Verification items for the finished model (mm, model axes). A direction names the side the tool comes from. Coordinates: 2 decimals unless noted, no trailing zeros. Order: outer loops, then holes, each group sorted by start corner. A loop starts at its lowest first (then second) coordinate and runs counter-clockwise, first axis right, second up. Notation, with made-up numbers: (57.5, 16) -> (81.5, 16) arc R19 ccw to (81.5, 34) -> close; hole circle Ø4 at (26, 38.5). An arc over 180 degrees is marked (long way). Answer as CSV lines item,"result".
```python
from build123d import *

# Parameters (mm, degrees)
EXTRUDE_1_DEPTH          = 5
SKETCH_2_W               = 4
SKETCH_2_H               = 40
EXTRUDE_2_DEPTH          = 36
EXTRUDE_3_DEPTH          = 7.5
CUT_EXTRUDE_2_DEPTH      = 14
EXTRUDE_START            = 18
SKETCH_5_W               = 5
SKETCH_5_H               = 27.5
EXTRUDE_4_DEPTH          = 18
SKETCH_6_R               = 15
SKETCH_6_R_2             = 1.5
CUT_EXTRUDE_3_DEPTH      = 18
CUT_EXTRUDE_4_DEPTH      = 15
CUT_EXTRUDE_4_DEPTH_BACK = 26
SKETCH_9_R               = 1.65
CUT_EXTRUDE_5_DEPTH      = 41
RIB_2_REACH              = 138.99
SKETCH_10_WALL_W         = 293.529278964
SKETCH_10_WALL_H         = 10
EXTRUDE_6_DEPTH          = 5
SKETCH_12_W              = 36
SKETCH_12_H              = 5
CUT_EXTRUDE_6_DEPTH      = 87


with BuildPart() as part:
    # 草图1 → 凸台-拉伸1 (new body)
    with BuildSketch(Plane.XY):
        with BuildLine():
            Line((105.214975384, -55), (105.214975384, 50))
            Line((105.214975384, 50), (-51, 50))
            ThreePointArc((-51, 50), (-53.828427125, 48.828427125), (-55, 46))
            Line((-55, 46), (-55, -46))
            ThreePointArc((-55, -46), (-53.828427125, -48.828427125), (-51, -50))
            Line((-51, -50), (-49.468062182, -50))
            Line((-49.468062182, -50), (-49.468062182, -55))
            Line((-49.468062182, -55), (-39.468062182, -55))
            Line((-39.468062182, -55), (-39.468062182, -50))
            Line((-39.468062182, -50), (35.214975384, -50))
            Line((35.214975384, -50), (35.214975384, -55))
            Line((35.214975384, -55), (105.214975384, -55))
        make_face()
    extrude(amount=EXTRUDE_1_DEPTH)

    # 草图2 → 凸台-拉伸2 (add)
    with BuildSketch(Plane(origin=(0, 0, 0), x_dir=(-1, 0, 0), z_dir=(0, 0, -1))):
        with Locations((35, 21.933022766)):
            Rectangle(SKETCH_2_W, SKETCH_2_H)
        with Locations((-1, 21.933022766)):
            Rectangle(SKETCH_2_W, SKETCH_2_H)
        with Locations((-18, 21.933022766)):
            Rectangle(SKETCH_2_W, SKETCH_2_H)
    extrude(amount=EXTRUDE_2_DEPTH)

    # 草图3 → 凸台-拉伸3 (add, symmetric)
    with BuildSketch(Plane(origin=(0, 20, 0), x_dir=(1, 0, 0), z_dir=(0, 1, 0))):
        Polygon((20, 12.468062182), (20, 0), (30.673808223, 0), align=None)
        Polygon((16, 12.468062182), (9.436406156, 0), (16, 0), align=None)
        Polygon((3, 12.468062182), (3, 0), (9.436406156, 0), align=None)
        Polygon((-1, 12.468062182), (-8.755927232, 0), (-1, 0), align=None)
        Polygon((-33, 12.468062182), (-33, 0), (-24.531937818, 0), align=None)
        Polygon((-37, 12.468062182), (-49.468062182, 0), (-37, 0), align=None)
    extrude(amount=EXTRUDE_3_DEPTH, both=True)

    # 草图4 → 切除-拉伸2 (cut)
    with BuildSketch(Plane(origin=(0, 0, 0), x_dir=(-1, 0, 0), z_dir=(0, 0, -1))):
        with BuildLine():
            Line((18.5, -18.5), (18.5, -36))
            ThreePointArc((18.5, -36), (19.671572875, -38.828427125), (22.5, -40))
            Line((22.5, -40), (48, -40))
            ThreePointArc((48, -40), (50.121320344, -39.121320344), (51, -37))
            Line((51, -37), (51, -17.5))
            ThreePointArc((51, -17.5), (50.121320344, -15.378679656), (48, -14.5))
            Line((48, -14.5), (22.5, -14.5))
            ThreePointArc((22.5, -14.5), (19.671572875, -15.671572875), (18.5, -18.5))
        make_face()
    extrude(amount=-CUT_EXTRUDE_2_DEPTH, mode=Mode.SUBTRACT)

    # 草图5 → 凸台-拉伸4 (add)
    with BuildSketch(Plane(origin=(0, 0, 0), x_dir=(-1, 0, 0), z_dir=(0, 0, -1)).offset(EXTRUDE_START)):
        with Locations((-43.5, -27.25)):
            Rectangle(SKETCH_5_W, SKETCH_5_H)
        with BuildLine():
            Line((18.5, -18.5), (18.5, -36))
            ThreePointArc((18.5, -36), (19.671572875, -38.828427125), (22.5, -40))
            Line((22.5, -40), (48, -40))
            Line((48, -40), (48, -44))
            Line((48, -44), (11.223006292, -44))
            Line((11.223006292, -44), (11.223006292, -41))
            Line((11.223006292, -41), (11.223006292, -13.5))
            Line((11.223006292, -13.5), (11.223006292, -10.5))
            Line((11.223006292, -10.5), (48, -10.5))
            Line((48, -10.5), (48, -14.5))
            Line((48, -14.5), (22.5, -14.5))
            ThreePointArc((22.5, -14.5), (19.671572875, -15.671572875), (18.5, -18.5))
        make_face()
    extrude(amount=-EXTRUDE_4_DEPTH)

    # 草图6 → 切除-拉伸3 (cut)
    with BuildSketch(Plane(origin=(0, 0, 0), x_dir=(-1, 0, 0), z_dir=(0, 0, -1))):
        with Locations((-11.776993708, -27.5)):
            Circle(SKETCH_6_R)
        with Locations((4.223006292, -43.5)):
            Circle(SKETCH_6_R_2)
        with Locations((4.223006292, -11.5)):
            Circle(SKETCH_6_R_2)
        with Locations((-27.776993708, -11.5)):
            Circle(SKETCH_6_R_2)
        with Locations((-27.776993708, -43.5)):
            Circle(SKETCH_6_R_2)
    extrude(amount=-CUT_EXTRUDE_3_DEPTH, mode=Mode.SUBTRACT)

    # 草图7 → 切除-拉伸4 (cut, two sides: drawn at the far end of the back side and taken through both)
    with BuildSketch(Plane.XY.offset(5).offset(-CUT_EXTRUDE_4_DEPTH_BACK)):
        with BuildLine():
            Line((78.295417345, 28.5), (87.295417345, 28.5))
            ThreePointArc((87.295417345, 28.5), (88.709630907, 29.085786438), (89.295417345, 30.5))
            Line((89.295417345, 30.5), (89.295417345, 32.5))
            ThreePointArc((89.295417345, 32.5), (88.709630907, 33.914213562), (87.295417345, 34.5))
            Line((87.295417345, 34.5), (78.295417345, 34.5))
            ThreePointArc((78.295417345, 34.5), (76.881203783, 33.914213562), (76.295417345, 32.5))
            Line((76.295417345, 32.5), (76.295417345, 30.5))
            ThreePointArc((76.295417345, 30.5), (76.881203783, 29.085786438), (78.295417345, 28.5))
        make_face()
    extrude(amount=CUT_EXTRUDE_4_DEPTH + CUT_EXTRUDE_4_DEPTH_BACK, mode=Mode.SUBTRACT)

    # 草图9 → 切除-拉伸5 (cut)
    with BuildSketch(Plane.XY.offset(5)):
        with Locations((-44.468062182, -50.360148647)):
            Circle(SKETCH_9_R)
        with Locations((-51.519821375, 46.879485601)):
            Circle(SKETCH_9_R)
        with Locations((60.214975384, -48.977955399)):
            Circle(SKETCH_9_R)
        with Locations((59.391625653, 46)):
            Circle(SKETCH_9_R)
        with Locations((98.214975384, -48.977955399)):
            Circle(SKETCH_9_R)
        with Locations((94.391625653, 46)):
            Circle(SKETCH_9_R)
    extrude(amount=-CUT_EXTRUDE_5_DEPTH, mode=Mode.SUBTRACT)

    # 草图10 wall → 筋2 (add, up to next)
    with BuildSketch(Plane(origin=(50.748705284, -30, -7.378924001), x_dir=(0.541169685132, 0, 0.840913415218), z_dir=(0.840913415218, 0, -0.541169685132)), mode=Mode.PRIVATE) as rib_2_sk1:
        Rectangle(SKETCH_10_WALL_W, SKETCH_10_WALL_H)
    rib_2_tool1 = extrude(rib_2_sk1.sketch, amount=-RIB_2_REACH, mode=Mode.PRIVATE) - part.part
    add(rib_2_tool1.solids().sort_by_distance((50.748705284, -30, -7.378924001))[0])

    # 草图11 → 凸台-拉伸6 (add)
    with BuildSketch(Plane(origin=(46, 0, 0), x_dir=(0, 0, -1), z_dir=(1, 0, 0))):
        Polygon((18, -13.5), (0, -4.773458624), (0, -13.5), align=None)
    extrude(amount=-EXTRUDE_6_DEPTH)

    # 草图12 → 切除-拉伸6 (cut)
    with BuildSketch(Plane(origin=(20, 0, 0), x_dir=(0, 0, -1), z_dir=(1, 0, 0))):
        with Locations((18, 4.433022766)):
            Rectangle(SKETCH_12_W, SKETCH_12_H)
    extrude(amount=-CUT_EXTRUDE_6_DEPTH, mode=Mode.SUBTRACT)


solid = part.part
```
Item 1: Section check C-C, the plane y = 9. Record the boundary of the cut face in (x, z).
Answer list:
outline,"(-55, 0) -> (-37, 0) -> (-37, -36) -> (-33, -36) -> (-33, 0) -> (-1, 0) -> (-1, -36) -> (3, -36) -> (3, 0) -> (16, 0) -> (16, -36) -> (20, -36) -> (20, 0) -> (105.21, 0) -> (105.21, 5) -> (-55, 5) -> close"
Item 2: Section check B-B, the plane x = 43. Record the boundary of the cut face in (y, z), plus the area to 3 significant figures.
Answer list:
outline,"(-55, 0) -> (-41, 0) -> (-41, -18) -> (-13.5, -18) -> (-4.77, 0) -> (50, 0) -> (50, 5) -> (-55, 5) -> close"
area,"1,100 mm2"
Item 3: Depth check by flat-ended pin: pin 1 Ø1.5 at (x, y) = (48.5, 0.5) entering from -Z; pin 2 Ø11.5 at (x, z) = (27, -5) entering from -Y; pin 3 Ø9 at (y, z) = (-30.5, -10) entering from +X; pin 4 Ø19 at (y, z) = (-27, -1.5) entering from -X. Enter the tip coordinate at first touch or a pass-through.
Answer list:
pin 1,"z = 0"
pin 2,"y = -50"
pin 3,"x = 51.96"
pin 4,"x = -55"
Item 4: Section check D-D, the plane x = 7. Record the boundary of the cut face in (y, z), plus the area to 3 significant figures.
Answer list:
outline,"(-50, 0) -> (-41.72, 0) -> (-41.72, 5) -> (-50, 5) -> close; (-13.28, 0) -> (12.5, 0) -> (12.5, -4.72) -> (27.5, -4.72) -> (27.5, 0) -> (50, 0) -> (50, 5) -> (-13.28, 5) -> close"
area,"429 mm2"
Item 5: Release check for a two-part mould opening along Y. For faces 1 (the flat face through (23, 12.5, -4)), 2 (the cylindrical face through (-19.641, -38.797, -6.661)), 3 (the flat face through (24, -2, 5)), 4 (the flat face through (23, 27.5, -4)) record: +Y half, -Y half, draft (parallel to the pull), parting line (faces both ways), or undercut.
Answer list:
face 1,"-Y half"
face 2,"undercut"
face 3,"draft"
face 4,"+Y half"
Item 6: Thickness scan on line 1 (X direction, y = 8.5, z = -4.5); line 2 (Y direction, x = -29.5, z = -11); line 3 (Y direction, x = -28, z = 1). Record the ranges inside material, lowest first.
Answer list:
line 1,"-37 to -33, -1 to 3, 16 to 20"
line 2,"-44 to -40, -14.5 to -10.5"
line 3,"-50 to -40, -14.5 to 50"
Item 7: Tool access check on faces 5 (the flat face through (43.54, -9.2, -9.13)), 6 (the flat face through (18, 41.933, -18)), 7 (the flat face through (6.26, 19.9, -6.15)), 8 (the cylindrical face through (-50.1, -39.14, 2.46)). Record the directions out of +Z, -Z, +X, -X, +Y, -Y that give a thin tool (end or side, any length) a straight path to the whole face; none if there is none.
Answer list:
face 5,"-Z, +X, +Y"
face 6,"-Z, +X, -X, +Y"
face 7,"-Z, +Y, -Y"
face 8,"+Z, -Z"
Item 8: Section check A-A, the plane y = -27.5. Record the boundary of the cut face in (x, z), plus the area to 3 significant figures.
Answer list:
outline,"(-55, 0) -> (-51, 0) -> (-51, 5) -> (-55, 5) -> close; (-18.5, -18) -> (-11.22, -18) -> (-11.22, 0) -> (-3.22, 0) -> (-3.22, 5) -> (-18.5, 5) -> close; (26.78, 0) -> (41, 0) -> (41, -18) -> (46, -18) -> (46, -14.76) -> (55.5, 0) -> (105.21, 0) -> (105.21, 5) -> (26.78, 5) -> close"
area,"780 mm2"
